Here's how the part is built. I have some questions about the finished solid (model axes, mm). Give positions to 0.01 mm unless a question says otherwise; leave off trailing zeros. Write each loop counter-clockwise with the first axis right and the second up, starting at its lowest first coordinate (ties: lowest second). Pieces come first, ordered by that corner, then holes. Notation, with made-up numbers: M 46,27 L 78,27 A24 ccw 78,48 Z; hole C -37,1.5 d1. An arc over 180 degrees is marked long. Answer as CSV lines item,"result". Start each with the question number.
Q1. Suppose I cut it at A-A (x = -76.2). Write out the boundary of the cut face in (y, z) (3 decimals), then the cut area to 3 significant figures.
Q2. For pin 1 (5 mm diameter, centred on x = 35, y = 28, fed in from +Z); pin 2 (12.5 mm diameter, centred on x = -76.2, y = 28.575, fed in from +Z), each with a flat end and sliding along its axis, tell me the tip position at first contact or that it passes through.
Q3. Suppose I cut it at C-C (x = 75). Write out the boundary of the cut face in (y, z) (3 decimals), then the cut area to 3 significant figures.
Q4. Suppose I cut it at B-B (z = 62.4). Write out the boundary of the cut face in (x, y) (3 decimals).
Q5. If I drill on line 1 along Y through (x, z) = (-25.4, 62.05); line 2 along X through (y, z) = (32.5, 61.9) (3 decimals); line 3 along X through (y, z) = (20.5, 60.6) (3 decimals), over which ranges is the centre line in solid material (lowest first)?
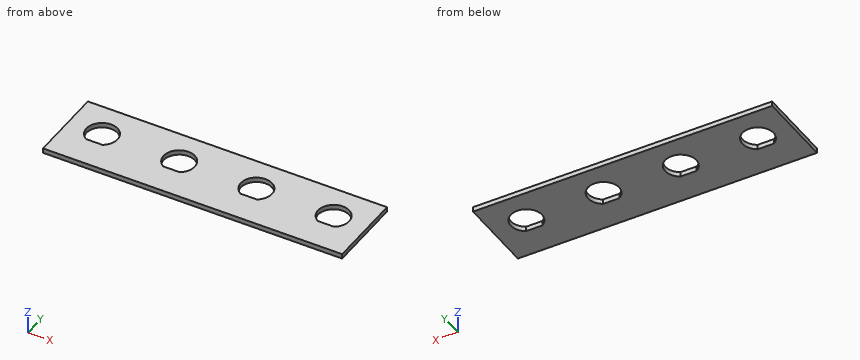
```python
from build123d import *

# Parameters (mm, degrees)
SKETCH1_W           = 203.2
SKETCH1_H           = 127
BOSS_EXTRUDE1_DEPTH = 50.8
SKETCH2_W           = 196.85
SKETCH2_H           = 120.65
CUT_EXTRUDE1_DEPTH  = 51.8
SKETCH4_W           = 203.2
SKETCH4_H           = 127
SKETCH4_W_2         = 196.85
SKETCH4_H_2         = 120.65
BOSS_EXTRUDE2_DEPTH = 6.35
CUT_EXTRUDE5_DEPTH  = 128
CUT_EXTRUDE6_REACH  = 205.2
CUT_EXTRUDE7_REACH  = 205.2
SKETCH13_R          = 12.55395
CUT_EXTRUDE8_DEPTH  = 51.8


with BuildPart() as part:
    # Sketch1 → Boss-Extrude1 (new body)
    with BuildSketch(Plane(origin=(0, 0, 0), x_dir=(1, 0, 0), z_dir=(0, 1, 0))):
        Rectangle(SKETCH1_W, SKETCH1_H)
    extrude(amount=BOSS_EXTRUDE1_DEPTH)

    # Sketch2 → Cut-Extrude1 (cut, through all)
    with BuildSketch(Plane(origin=(0, 50.8, 0), x_dir=(1, 0, 0), z_dir=(0, 1, 0))):
        Rectangle(SKETCH2_W, SKETCH2_H)
    extrude(amount=-CUT_EXTRUDE1_DEPTH, mode=Mode.SUBTRACT)

    # Sketch4 → Boss-Extrude2 (add)
    with BuildSketch(Plane(origin=(0, 50.8, 0), x_dir=(1, 0, 0), z_dir=(0, 1, 0))):
        Rectangle(SKETCH4_W, SKETCH4_H)
        Rectangle(SKETCH4_W_2, SKETCH4_H_2, mode=Mode.SUBTRACT)
    extrude(amount=-BOSS_EXTRUDE2_DEPTH)

    # Sketch10 → Cut-Extrude5 (cut, through all)
    with BuildSketch(Plane.XY.offset(63.5)):
        with BuildLine():
            ThreePointArc((-70.843294161, 19.8374), (-76.2, 38.8239), (-81.556705839, 19.8374))
            Line((-81.556705839, 19.8374), (-70.843294161, 19.8374))
        make_face()
        with BuildLine():
            ThreePointArc((81.556705839, 19.8374), (76.2, 38.8239), (70.843294161, 19.8374))
            Line((70.843294161, 19.8374), (81.556705839, 19.8374))
        make_face()
        with BuildLine():
            ThreePointArc((30.756705839, 19.8374), (25.4, 38.8239), (20.043294161, 19.8374))
            Line((20.043294161, 19.8374), (30.756705839, 19.8374))
        make_face()
        with BuildLine():
            ThreePointArc((-20.043294161, 19.8374), (-25.4, 38.8239), (-30.756705839, 19.8374))
            Line((-30.756705839, 19.8374), (-20.043294161, 19.8374))
        make_face()
    extrude(amount=-CUT_EXTRUDE5_DEPTH, mode=Mode.SUBTRACT)

    # Sketch12 → Cut-Extrude6 (cut, up to next)
    with BuildSketch(Plane(origin=(101.6, 0, 0), x_dir=(0, 0, -1), z_dir=(1, 0, 0)), mode=Mode.PRIVATE) as cut_extrude6_sk1:
        with BuildLine():
            ThreePointArc((-20.043294161, 19.8374), (-25.4, 38.8239), (-30.756705839, 19.8374))
            Line((-30.756705839, 19.8374), (-20.043294161, 19.8374))
        make_face()
    cut_extrude6_tool1 = extrude(cut_extrude6_sk1.sketch, amount=-CUT_EXTRUDE6_REACH, mode=Mode.PRIVATE) & part.part
    add(cut_extrude6_tool1.solids().sort_by_distance((101.6, 28.896198, 25.4))[0], mode=Mode.SUBTRACT)
    # Sketch12 → Cut-Extrude6 (cut, up to next)
    with BuildSketch(Plane(origin=(101.6, 0, 0), x_dir=(0, 0, -1), z_dir=(1, 0, 0)), mode=Mode.PRIVATE) as cut_extrude6_sk2:
        with BuildLine():
            ThreePointArc((30.756705839, 19.8374), (25.4, 38.8239), (20.043294161, 19.8374))
            Line((20.043294161, 19.8374), (30.756705839, 19.8374))
        make_face()
    cut_extrude6_tool2 = extrude(cut_extrude6_sk2.sketch, amount=-CUT_EXTRUDE6_REACH, mode=Mode.PRIVATE) & part.part
    add(cut_extrude6_tool2.solids().sort_by_distance((101.6, 28.896198, -25.4))[0], mode=Mode.SUBTRACT)

    # Sketch13 → Cut-Extrude7 (cut, up to next)
    with BuildSketch(Plane.ZY.offset(101.6), mode=Mode.PRIVATE) as cut_extrude7_sk1:
        with Locations((12.7, 28.575)):
            Circle(SKETCH13_R)
    cut_extrude7_tool1 = extrude(cut_extrude7_sk1.sketch, amount=-CUT_EXTRUDE7_REACH, mode=Mode.PRIVATE) & part.part
    add(cut_extrude7_tool1.solids().sort_by_distance((-101.6, 28.575, 12.7))[0], mode=Mode.SUBTRACT)

    # Sketch14 → Cut-Extrude8 (cut, through all)
    with BuildSketch(Plane(origin=(0, 50.8, 0), x_dir=(1, 0, 0), z_dir=(0, 1, 0))):
        Polygon((-98.425, -60.325), (-98.425, -63.5), (-101.6, -63.5), (-101.6, 63.5), (101.6, 63.5), (101.6, -63.5), (98.425, -63.5), (98.425, -60.325), align=None)
    extrude(amount=-CUT_EXTRUDE8_DEPTH, mode=Mode.SUBTRACT)


solid = part.part
```
Resolved:
1,outline,"M 0,60.325 L 19.837,60.325 L 19.837,63.5 L 0,63.5 Z; M 38.824,60.325 L 50.8,60.325 L 50.8,63.5 L 38.824,63.5 Z"
1,area,"101 mm^2"
2,pin 1,"z = 63.5"
2,pin 2,"through"
3,outline,"M 0,60.325 L 19.837,60.325 L 19.837,63.5 L 0,63.5 Z; M 38.753,60.325 L 50.8,60.325 L 50.8,63.5 L 38.753,63.5 Z"
3,area,"101 mm^2"
4,outline,"M -98.425,0 L 98.425,0 L 98.425,50.8 L -98.425,50.8 Z; hole M -81.557,19.837 L -70.843,19.837 A10.249 ccw long Z; hole M -30.757,19.837 L -20.043,19.837 A10.249 ccw long Z; hole M 20.043,19.837 L 30.757,19.837 A10.249 ccw long Z; hole M 70.843,19.837 L 81.557,19.837 A10.249 ccw long Z"
5,line 1,"0 to 19.84, 38.82 to 50.8"
5,line 2,"-98.425 to -85.668, -66.732 to -34.868, -15.932 to 15.932, 34.868 to 66.732, 85.668 to 98.425"
5,line 3,"-98.425 to -82.511, -69.889 to -31.711, -19.089 to 19.089, 31.711 to 69.889, 82.511 to 98.425"
